Study the drawing (mm; zero at the part's minimum x, y, z) and answer. A direction names the side the tool comes from. Coordinates: 2 decimals unless noted, no trailing zeros. Order: outer loops, then holes, each group sorted by start corner. A loop starts at its lowest first (then second) coordinate and runs counter-clockwise, first axis right, second up. Notation, with made-up numbers: M 64,66 L 107,66 A21 cw 107,100 Z; hole C 11,24 d6. An arc over 180 degrees is marked long. Use a Markdown table: item, result. Add a question column.
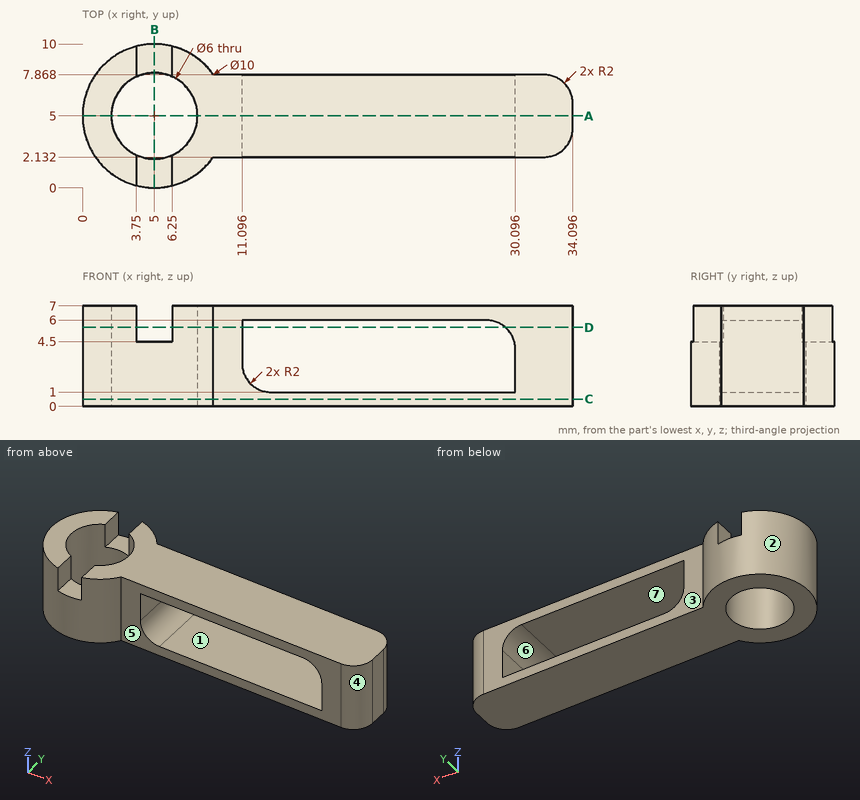
(1) Straight lines are drawn through the part: line 1 (X direction, y = 5, z = 3); line 2 (X direction, y = 5, z = 5) (1 decimal); line 3 (Z direction, x = 13, y = 5.75). For each, find the intervals that lie inside material, in ascending order.
(2) A cutting plane is placed at D-D on z = 5.5. Write down the section's boundary in (x, y).
(3) A cutting plane is placed at C-C on z = 0.5. Write down the section's boundary in (x, y).
(4) A cutting plane is placed at B-B on x = 5. Write down the section's boundary in (y, z).
(5) A cutting plane is placed at A-A on y = 5. Write down the section's boundary in (x, z).
(6) Given P1, Ø3.5, axis at x = 23.5, z = 3.5, coming from the -Y side; P2, Ø1.5, axis at x = 7.5, z = 5.5, coming from the +Y side; P3, Ø2.5, axis at y = 1.5, z = 6, coming from the +X side; P4, Ø0.6, axis at y = 1.5, z = 5.5, coming from the -X side, each flat-ended and moving along its own axis, determine where each tip first touches the part or whether it passes through.
(7) The mould has two halves that part along X. Classify the marked faces 4, 5, 6 and 7: pulls with the +X half, pulls with the -X half, needs draft (parallel to the pull), parting line crosses it, or undercut.
(8) Which of the six approach directions +Z, -Z, +X, -X, +Y, -Y give full straight-line access (tool end or side, diameter ignored) to the marked faces 1, 2 and 3?
From the geometry:
| question | item | result |
|---|---|---|
| 1 | line 1 | x = 0 to 2, 8 to 11.1, 30.1 to 34.1 |
| 1 | line 2 | x = 0 to 2, 8 to 11.1, 29.8 to 34.1 |
| 1 | line 3 | z = 0 to 1, 6 to 7 |
| 2 | outline | M 3.75,0.16 L 3.75,2.27 A3 cw 3.75,7.73 L 3.75,9.84 A5 ccw Z; M 6.25,0.16 A5 ccw 9.1,2.13 L 11.1,2.13 L 11.1,7.87 L 9.1,7.87 A5 ccw 6.25,9.84 L 6.25,7.73 A3 cw 6.25,2.27 Z; M 29.42,2.13 L 32.1,2.13 A2 ccw 34.1,4.13 L 34.1,5.87 A2 ccw 32.1,7.87 L 29.42,7.87 Z |
| 3 | outline | M 9.1,2.13 L 32.1,2.13 A2 ccw 34.1,4.13 L 34.1,5.87 A2 ccw 32.1,7.87 L 9.1,7.87 A5 ccw long Z; hole C 5,5 d6 |
| 4 | outline | M 0,0 L 2,0 L 2,4.5 L 0,4.5 Z; M 8,0 L 10,0 L 10,4.5 L 8,4.5 Z |
| 5 | outline | M 0,0 L 2,0 L 2,7 L 0,7 Z; M 8,0 L 34.1,0 L 34.1,7 L 8,7 Z; hole M 11.1,3 A2 ccw 13.1,1 L 30.1,1 L 30.1,4 A2 ccw 28.1,6 L 11.1,6 Z |
| 6 | P1 | passes through |
| 6 | P2 | stops at y = 9.68 |
| 6 | P3 | stops at x = 33.54 |
| 6 | P4 | stops at x = 1.16 |
| 7 | face 4 | pulls with the +X half |
| 7 | face 5 | needs draft |
| 7 | face 6 | undercut |
| 7 | face 7 | undercut |
| 8 | face 1 | +Y, -Y |
| 8 | face 2 | +Z, -Z |
| 8 | face 3 | +Z, -Z, +X, +Y |
